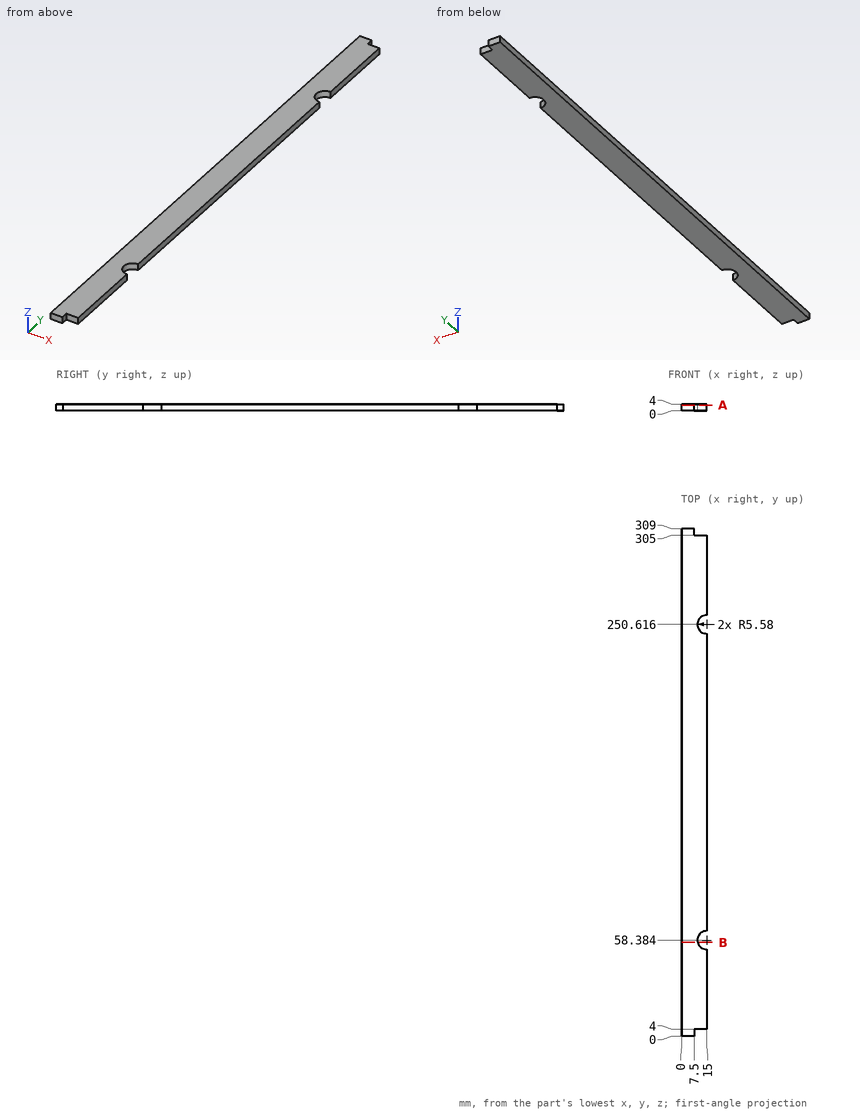
Study the drawing (mm; zero at the part's minimum x, y, z) and answer. Round coordinates to 2 decimals unless told otherwise and drop trailing zeros. Write each loop counter-clockwise with the first axis right and the second up, starting at its lowest first coordinate (ties: lowest second). Pieces come first, ordered by that corner, then holes.
1) Straight lines are drawn through the part: line 1 (Y direction, x = 10.25, z = 1.7) (1 decimal); line 2 (Y direction, x = 13, z = 2) (1 decimal); line 3 (Y direction, x = 7.75, z = 0.8). For each, find the intervals that lie inside material, in ascending order.
2) A cutting plane is placed at A-A (z = 3.3). Give the vertices of the cut face in (x, y) (1 decimal).
3) A cutting plane is placed at B-B (y = 57). Give the vertices of the cut face in (x, z) (1 decimal), plus the area to 3 significant figures.
4) Given pin 1 Ø1.2 at (x, z) = (12, 1.5) entering from +Y; pin 2 Ø1.2 at (y, z) = (2, 1.5) entering from +X; pin 3 Ø1.2 at (x, z) = (11.5, 1.5) entering from -Y, each flat-ended and moving along its own axis, determine where each tip first touches the part or whether it passes through.
Completed:
1. line 1: y = 4 to 55.5, 61.3 to 247.7, 253.5 to 305
1. line 2: y = 4 to 53.2, 63.6 to 245.4, 255.8 to 305
1. line 3: y = 4 to 305
2. outline: (0, 0) - (7.5, 0) - (7.5, 4) - (15, 4) - (15, 52.8) arc R5.6 cw to (15, 64) - (15, 245) arc R5.6 cw to (15, 256.2) - (15, 305) - (7.5, 305) - (7.5, 309) - (0, 309) - close
3. outline: (0, 0) - (9.6, 0) - (9.6, 4) - (0, 4) - close
3. area: 38.4 mm2
4. pin 1: stops at y = 305
4. pin 2: stops at x = 7.5
4. pin 3: stops at y = 4
